Input: part model. Units: mm. Frame: model coordinates. Give positions to 0.01 mm unless a question says otherwise; leave off trailing zeros. Order: outer loops, then holes, each group sorted by start corner. A loop starts at its lowest first (then second) coordinate and runs counter-clockwise, first axis right, second up. Notation, with made-up numbers: (-1, 29.5) - (25, 29.5) arc R22 cw to (25, 45.5) - close; hole circle Ø10 at (0, 13). An arc over 180 degrees is marked (long way). Use a Markdown table: item, result.
Autodesk Inventor part; units mm, degrees
ref_plane "YZ Plane" through (0, 0, 0) normal (1, 0, 0) x (0, 1, 0)
ref_plane "XZ Plane" through (0, 0, 0) normal (0, 1, 0) x (-1, 0, 0)
ref_plane "XY Plane" through (0, 0, 0) normal (0, 0, 1) x (1, 0, 0)
sketch "Sketch2" plane through (0, 0, 0) normal (0, 0, 1) x (1, 0, 0)
  arc A0 (-32, 4) -> (-32, -4) centre (-32, 0) ccw
  arc A1 (32, -4) -> (32, 4) centre (32, 0) ccw
  line L0 (-32, 4) -> (32, 4)
  line L1 (-32, -4) -> (32, -4)
  line L2 (-50.4, 0) -> (50.4, 0)
  line L3 (0, -5.6) -> (0, 5.6)
  point P0 (0, 0)
  dimension "d0" = 4
  dimension "d1" = 4
  dimension "d2" = 64
  dimension "d3" = 0
  dimension "d4" = 32
  dimension "d9" = 180
  dimension "d10" = 0
  dimension "d141" = 64
extrude "Extrusion1" add sketch "Sketch2" along normal blind 8
sketch "Sketch15" plane through (0, 0, 8) normal (0, 0, 1) x (1, 0, 0)
  arc A0 (-32, 4) -> (-32, -4) centre (-32, 0) ccw
  circle A1 centre (-32, 0) radius 2.5
  line L0 (-50.4, 0) -> (50.4, 0)
  circle A2 centre (-24, 0) radius 2.5
  circle A3 centre (-16, 0) radius 2.5
  circle A4 centre (-8, 0) radius 2.5
  circle A5 centre (0, 0) radius 2.5
  circle A6 centre (8, 0) radius 2.5
  circle A7 centre (16, 0) radius 2.5
  circle A8 centre (24, 0) radius 2.5
  circle A9 centre (32, 0) radius 2.5
  dimension "d142" = 5
  dimension "d148" = 8
extrude "Extrusion14" cut sketch "Sketch15" against normal through all
sketch "Sketch16" plane through (0, 0, 8) normal (0, 0, 1) x (1, 0, 0)
  circle A0 centre (32, 0) radius 2.5
  circle A1 centre (24, 0) radius 2.5
  circle A2 centre (16, 0) radius 2.5
  circle A3 centre (8, 0) radius 2.5
  circle A4 centre (0, 0) radius 2.5
  circle A5 centre (-8, 0) radius 2.5
  circle A6 centre (-16, 0) radius 2.5
  circle A7 centre (-24, 0) radius 2.5
  circle A8 centre (-32, 0) radius 2.5
  arc A9 (-32, 4) -> (-32, -4) centre (-32, 0) ccw
  circle A10 centre (-32, 0) radius 3
  line L0 (-50.4, 0) -> (50.4, 0)
  circle A11 centre (-24, 0) radius 3
  circle A12 centre (-16, 0) radius 3
  circle A13 centre (-8, 0) radius 3
  circle A14 centre (0, 0) radius 3
  circle A15 centre (8, 0) radius 3
  circle A16 centre (16, 0) radius 3
  circle A17 centre (24, 0) radius 3
  circle A18 centre (32, 0) radius 3
  dimension "d152" = 6
  dimension "d158" = 8
extrude "Extrusion15" cut sketch "Sketch16" against normal blind 0.8 contours L0 A18 A0 | A0 L0 A18 | A10 L0 A8 | L0 A8 A10 | A11 L0 A7 | L0 A7 A11 | A12 L0 A6 | L0 A6 A12 | A13 L0 A5 | L0 A5 A13 | A14 L0 A4 | L0 A4 A14 | A15 L0 A3 | L0 A3 A15 | A16 L0 A2 | L0 A2 A16 | A17 L0 A1 | L0 A1 A17
sketch "Sketch17" plane through (0, 0, 0) normal (0, 0, -1) x (-1, 0, 0)
  circle A0 centre (-32, 0) radius 2.5
  circle A1 centre (-24, 0) radius 2.5
  circle A2 centre (-16, 0) radius 2.5
  circle A3 centre (-8, 0) radius 2.5
  circle A4 centre (0, 0) radius 2.5
  circle A5 centre (8, 0) radius 2.5
  circle A6 centre (16, 0) radius 2.5
  circle A7 centre (24, 0) radius 2.5
  circle A8 centre (32, 0) radius 2.5
  arc A9 (-32, 4) -> (-32, -4) centre (-32, 0) ccw
  circle A10 centre (-32, 0) radius 3
  line L0 (50.4, 0) -> (-50.4, 0)
  circle A11 centre (-24, 0) radius 3
  circle A12 centre (-16, 0) radius 3
  circle A13 centre (-8, 0) radius 3
  circle A14 centre (0, 0) radius 3
  circle A15 centre (8, 0) radius 3
  circle A16 centre (16, 0) radius 3
  circle A17 centre (24, 0) radius 3
  circle A18 centre (32, 0) radius 3
  dimension "d162" = 6
  dimension "d168" = 8
extrude "Extrusion16" cut sketch "Sketch17" against normal blind 0.8 contours L0 A10 A0 | A0 L0 A10 | A18 L0 A8 | L0 A8 A18 | A17 L0 A7 | L0 A7 A17 | A16 L0 A6 | L0 A6 A16 | A15 L0 A5 | L0 A5 A15 | A14 L0 A4 | L0 A4 A14 | A13 L0 A3 | L0 A3 A13 | A12 L0 A2 | L0 A2 A12 | A11 L0 A1 | L0 A1 A11
sketch "Sketch18" plane through (0, 0, 8) normal (0, 0, 1) x (1, 0, 0)
  circle A0 centre (-32, 0) radius 3
  circle A1 centre (-24, 0) radius 3
  arc A2 (-32, 4) -> (-32, -4) centre (-32, 0) ccw
  line L0 (-32, 4) -> (32, 4)
  arc A3 (-30.1972, -3) -> (-30.1972, 3) centre (-32, 0) ccw
  arc A4 (-25.8028, 3) -> (-25.8028, -3) centre (-24, 0) ccw
  line L1 (-30.1972, 3) -> (-25.8028, 3)
  line L2 (-25.8028, -3) -> (-30.1972, -3)
  line L3 (-50.4, 0) -> (50.4, 0)
  arc A5 (-22.1972, -3) -> (-22.1972, 3) centre (-24, 0) ccw
  arc A6 (-17.8028, 3) -> (-17.8028, -3) centre (-16, 0) ccw
  line L4 (-22.1972, 3) -> (-17.8028, 3)
  line L5 (-17.8028, -3) -> (-22.1972, -3)
  arc A7 (-14.1972, -3) -> (-14.1972, 3) centre (-16, 0) ccw
  arc A8 (-9.8028, 3) -> (-9.8028, -3) centre (-8, 0) ccw
  line L6 (-14.1972, 3) -> (-9.8028, 3)
  line L7 (-9.8028, -3) -> (-14.1972, -3)
  arc A9 (-6.1972, -3) -> (-6.1972, 3) centre (-8, 0) ccw
  arc A10 (-1.8028, 3) -> (-1.8028, -3) centre (0, 0) ccw
  line L8 (-6.1972, 3) -> (-1.8028, 3)
  line L9 (-1.8028, -3) -> (-6.1972, -3)
  arc A11 (1.8028, -3) -> (1.8028, 3) centre (0, 0) ccw
  arc A12 (6.1972, 3) -> (6.1972, -3) centre (8, 0) ccw
  line L10 (1.8028, 3) -> (6.1972, 3)
  line L11 (6.1972, -3) -> (1.8028, -3)
  arc A13 (9.8028, -3) -> (9.8028, 3) centre (8, 0) ccw
  arc A14 (14.1972, 3) -> (14.1972, -3) centre (16, 0) ccw
  line L12 (9.8028, 3) -> (14.1972, 3)
  line L13 (14.1972, -3) -> (9.8028, -3)
  arc A15 (17.8028, -3) -> (17.8028, 3) centre (16, 0) ccw
  arc A16 (22.1972, 3) -> (22.1972, -3) centre (24, 0) ccw
  line L14 (17.8028, 3) -> (22.1972, 3)
  line L15 (22.1972, -3) -> (17.8028, -3)
  arc A17 (25.8028, -3) -> (25.8028, 3) centre (24, 0) ccw
  arc A18 (30.1972, 3) -> (30.1972, -3) centre (32, 0) ccw
  line L16 (25.8028, 3) -> (30.1972, 3)
  line L17 (30.1972, -3) -> (25.8028, -3)
  dimension "d172" = 7
  dimension "d173" = 7
  dimension "d179" = 8
extrude "Extrusion17" cut sketch "Sketch18" against normal through all contours A17 L16 A18 L3 | L3 A18 L17 A17 | A15 L14 A16 L3 | L3 A16 L15 A15 | A13 L12 A14 L3 | L3 A14 L13 A13 | A11 L10 A12 L3 | L3 A12 L11 A11 | A9 L8 A10 L3 | L3 A10 L9 A9 | A7 L6 A8 L3 | L3 A8 L7 A7 | A5 L4 A6 L3 | L3 A6 L5 A5 | A3 L1 A4 L3 | L3 A4 L2 A3
properties part number "9M Beam"
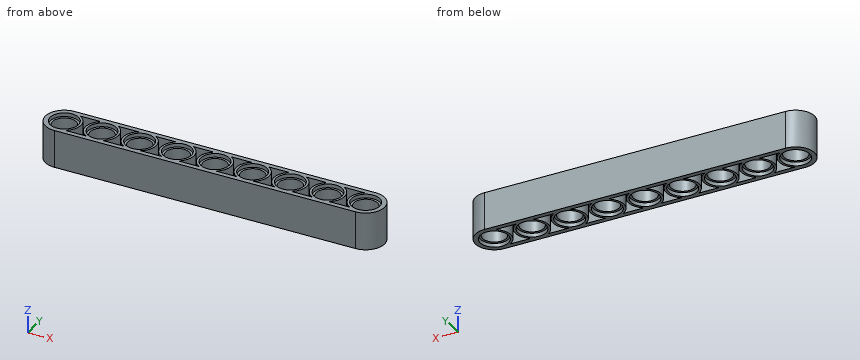
1. Pin query (flat end, axial travel): pin 1 (3.5 mm diameter, centred on x = 8, y = 0, fed in from +Z). Return the tip coordinate at first contact, or that it passes through.
Response:
| item | result |
|---|---|
| pin 1 | passes through |
2. Material intervals for line 1 along Y through (x, z) = (-27, 1); line 2 along Y through (x, z) = (-8, 7.8); line 3 along Y through (x, z) = (0, 4.75), sorted ascending.
Response:
| item | result |
|---|---|
| line 1 | y = -4 to -3, -1.8 to 1.8, 3 to 4 |
| line 2 | y = -4 to -3, 3 to 4 |
| line 3 | y = -4 to -2.5, 2.5 to 4 |
3. Section query B-B (z = 4.25). State how many separate pieces and enclosed holes the cut face has, then the cut area to 3 significant figures.
Response:
| item | result |
|---|---|
| separate pieces | 1 |
| enclosed holes | 17 |
| area | 290 mm^2 |
4. Section query A-A (x = 16). Return loops of the section in (y, z).
Response:
| item | result |
|---|---|
| outline | (-4, 0) - (-3, 0) - (-3, 0.8) - (-2.5, 0.8) - (-2.5, 7.2) - (-3, 7.2) - (-3, 8) - (-4, 8) - close; (2.5, 0.8) - (3, 0.8) - (3, 0) - (4, 0) - (4, 8) - (3, 8) - (3, 7.2) - (2.5, 7.2) - close |
